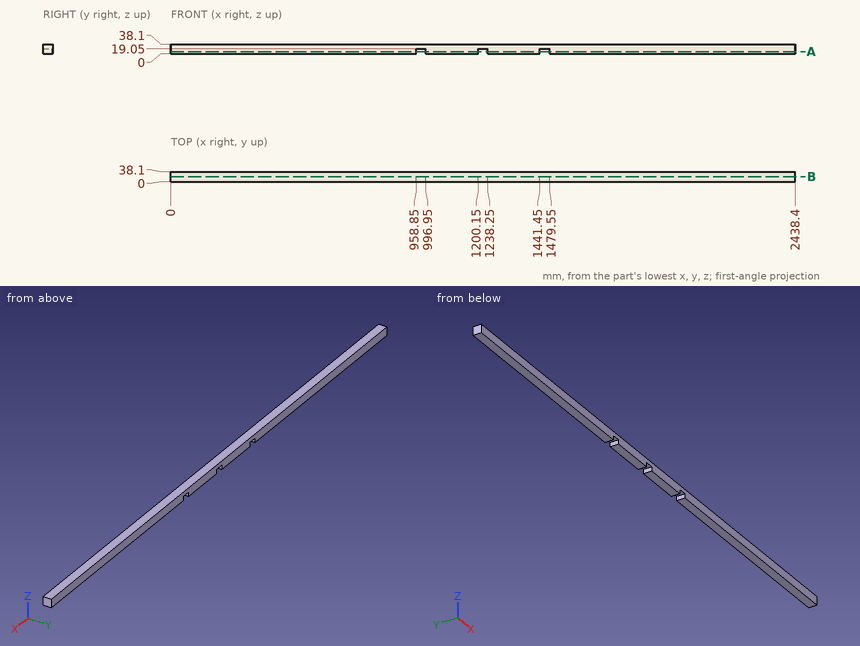
Geometry: see drawing. Coordinates: mm, zero at the bounding-box minimum. Give positions to 0.01 mm unless a question says otherwise; leave off trailing zeros. Order: outer loops, then holes, each group sorted by start corner. A loop starts at its lowest first (then second) coordinate and runs counter-clockwise, first axis right, second up.
Q1. Section A-A on z = 8.5. Output: boundary loops of the cut face in (x, y), and give its area (3 significant figures).
Checked values:
outline: (0, 0) - (958.85, 0) - (958.85, 38.1) - (0, 38.1) - close; (996.95, 0) - (1200.15, 0) - (1200.15, 38.1) - (996.95, 38.1) - close; (1238.25, 0) - (1441.45, 0) - (1441.45, 38.1) - (1238.25, 38.1) - close; (1479.55, 0) - (2438.4, 0) - (2438.4, 38.1) - (1479.55, 38.1) - close
area: 88,500 mm2
Q2. Contact query for a flat-ended pin moving along its axis: pin 1 Ø1.5 at (x, y) = (1475, 12.5) entering from -Z. Output: stop coordinate, or through.
Checked values:
pin 1: stops at z = 19.05
Q3. Section B-B on y = 19. Output: boundary loops of the cut face in (x, z).
Checked values:
outline: (0, 0) - (958.85, 0) - (958.85, 19.05) - (996.95, 19.05) - (996.95, 0) - (1200.15, 0) - (1200.15, 19.05) - (1238.25, 19.05) - (1238.25, 0) - (1441.45, 0) - (1441.45, 19.05) - (1479.55, 19.05) - (1479.55, 0) - (2438.4, 0) - (2438.4, 38.1) - (0, 38.1) - close
Q4. Ray query, probe 1 along X at (y, z) = (8.5, 18.5). Return the intervals inside material, ascending.
Checked values:
probe 1: x = 0 to 958.85, 996.95 to 1200.15, 1238.25 to 1441.45, 1479.55 to 2438.4
